Check sheet for the modelled part. Datum: model origin and axes. Units: mm. A direction names the side the tool comes from. Give positions to 0.01 mm unless a question says otherwise; leave off trailing zeros. Loops run counter-clockwise (first coordinate to the right, second up) from the corner with the lowest first, then second, coordinate; pieces in that order, holes last. Notation, with made-up numbers: (65, 22.25) - (110, 22.25) arc R20 ccw to (110, 34.25) - close; hole circle Ø11 at (-35.75, 73). An arc over 180 degrees is marked (long way). Use one line per item in the form item = value.
from build123d import *

# Parameters (mm, degrees)
F0_W     = 406.4
F0_H     = 406.4
F0_R     = 31.75
F1_DEPTH = 127
F2_W     = 381
F2_H     = 381
F2_R     = 31.75
F3_DEPTH = 101.6


with BuildPart() as f1:
    # F0 (on Top) → F1 (new body)
    with BuildSketch(Plane.XY):
        Rectangle(F0_W, F0_H)
        Circle(F0_R, mode=Mode.SUBTRACT)
    extrude(amount=F1_DEPTH)

    # F2 (on face) → F3 (cut)
    with BuildSketch(Plane.XY.offset(127)):
        Rectangle(F2_W, F2_H)
        Circle(F2_R, mode=Mode.SUBTRACT)
    extrude(amount=-F3_DEPTH, mode=Mode.SUBTRACT)


solid = f1.part
Item 1: Gauge pin test, flat end, axial feed: P1, Ø10, axis at x = -80, y = -73, coming from the +Z side. Record the tip position at first contact, or that the pin passes through.
Answer block:
P1 = 25.4
Item 2: Mould release check, pull along Y, two halves, no side actions. Record for faces 1 (the face through (40, 3, 25.4)), 2 (the face through (-3, 203.2, 63)), 3 (the face through (-3, -190.5, 77)), 4 (the face through (42, 3, 0)): released by +Y, released by -Y, zero draft, split by the parting line, or undercut.
Answer block:
face_1 = undercut
face_2 = released by +Y
face_3 = undercut
face_4 = zero draft
Item 3: Thickness scan on L1, parallel to Y at x = 172.5, z = 112; L2, parallel to Y at x = 0, z = 6. Record the ranges inside material, lowest first.
Answer block:
L1 = -203.2 to -190.5, 190.5 to 203.2
L2 = -203.2 to -31.75, 31.75 to 203.2
Item 4: Access from +Z, -Z, +X, -X, +Y, -Y to the whole of each face (thin tool, end or side, straight path). Record for faces 5 (the face through (-3, 190.5, 77)), 6 (the face through (-203.2, -3, 63)).
Answer block:
face_5 = +Z
face_6 = +Z, -Z, -X, +Y, -Y
Item 5: Section check D-D on y = 160.5. Record the boundary of the cut face in (x, z).
Answer block:
outline = (-203.2, 0) - (203.2, 0) - (203.2, 127) - (190.5, 127) - (190.5, 25.4) - (-190.5, 25.4) - (-190.5, 127) - (-203.2, 127) - close
Item 6: Section check A-A on y = 0. Record the boundary of the cut face in (x, z).
Answer block:
outline = (-203.2, 0) - (-31.75, 0) - (-31.75, 25.4) - (-190.5, 25.4) - (-190.5, 127) - (-203.2, 127) - close; (31.75, 0) - (203.2, 0) - (203.2, 127) - (190.5, 127) - (190.5, 25.4) - (31.75, 25.4) - close
Item 7: Section check C-C on z = 15. Record the boundary of the cut face in (x, y).
Answer block:
outline = (-203.2, -203.2) - (203.2, -203.2) - (203.2, 203.2) - (-203.2, 203.2) - close; hole circle Ø63.5 at (0, 0)
